```python
from build123d import *

# Parameters (mm, degrees)
SKETCH1_R           = 15.24
SKETCH1_R_2         = 4.55
BOSS_EXTRUDE1_DEPTH = 2.54
SKETCH2_R           = 5.95
BOSS_EXTRUDE2_DEPTH = 7
BOSS_EXTRUDE3_DEPTH = 38.1
SKETCH5_R           = 0.9525
BOSS_EXTRUDE5_DEPTH = 2.54


with BuildPart() as part:
    # Sketch1 → Boss-Extrude1 (new body)
    with BuildSketch(Plane.XY):
        Circle(SKETCH1_R)
        Circle(SKETCH1_R_2, mode=Mode.SUBTRACT)
    extrude(amount=BOSS_EXTRUDE1_DEPTH)

    # Sketch2 → Boss-Extrude2 (add)
    with BuildSketch(Plane.XY.offset(2.54)):
        Circle(SKETCH2_R)
    extrude(amount=BOSS_EXTRUDE2_DEPTH)

    # Sketch3 → Boss-Extrude3 (add)
    with BuildSketch(Plane.XY.offset(9.54)):
        Polygon((3.666174209, 6.35), (-3.666174209, 6.35), (-7.332348419, 0), (-3.666174209, -6.35), (3.666174209, -6.35), (7.332348419, 0), align=None)
    extrude(amount=BOSS_EXTRUDE3_DEPTH)

    # Sketch5 → Boss-Extrude5 (add)
    with BuildSketch(Plane(origin=(0, 0, 0), x_dir=(-1, 0, 0), z_dir=(0, 0, -1))):
        with Locations(Location((0, 12.7, 0), (0, 0, 180))):
            Circle(SKETCH5_R)
        with Locations(Location((5.165555367, 11.602027312, 0), (0, 0, 180))):
            Circle(SKETCH5_R)
        with Locations(Location((9.437939284, 8.497958701, 0), (0, 0, 180))):
            Circle(SKETCH5_R)
        with Locations(Location((12.078417757, 3.924515829, 0), (0, 0, 180))):
            Circle(SKETCH5_R)
        with Locations(Location((12.630428071, -1.327511483, 0), (0, 0, 180))):
            Circle(SKETCH5_R)
        with Locations(Location((10.998522628, -6.35, 0), (0, 0, 180))):
            Circle(SKETCH5_R)
        with Locations(Location((7.464872704, -10.274515829, 0), (0, 0, 180))):
            Circle(SKETCH5_R)
        with Locations(Location((2.640478473, -12.422474529, 0), (0, 0, 180))):
            Circle(SKETCH5_R)
        with Locations(Location((-2.640478473, -12.422474529, 0), (0, 0, 180))):
            Circle(SKETCH5_R)
        with Locations(Location((-7.464872704, -10.274515829, 0), (0, 0, 180))):
            Circle(SKETCH5_R)
        with Locations(Location((-10.998522628, -6.35, 0), (0, 0, 180))):
            Circle(SKETCH5_R)
        with Locations(Location((-12.630428071, -1.327511483, 0), (0, 0, 180))):
            Circle(SKETCH5_R)
        with Locations(Location((-12.078417757, 3.924515829, 0), (0, 0, 180))):
            Circle(SKETCH5_R)
        with Locations(Location((-9.437939284, 8.497958701, 0), (0, 0, 180))):
            Circle(SKETCH5_R)
        with Locations(Location((-5.165555367, 11.602027312, 0), (0, 0, 180))):
            Circle(SKETCH5_R)
    extrude(amount=BOSS_EXTRUDE5_DEPTH)


solid = part.part
```
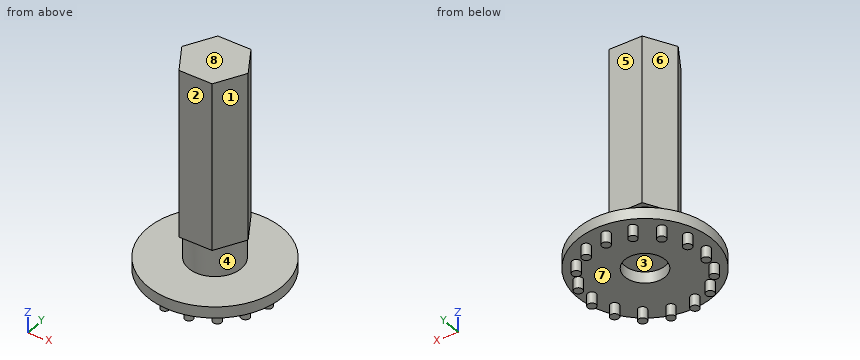
The model under review builds one solid part; all positions refer to its coordinate system, in mm. Face numbers are marked on the shaded views. A direction names the side the tool comes from. Round coordinates to 2 decimals unless told otherwise and drop trailing zeros. Loops run counter-clockwise (first coordinate to the right, second up) from the corner with the lowest first, then second, coordinate; pieces in that order, holes last. Notation, with made-up numbers: (35.25, 22) -> (52.25, 22) arc R15 cw to (52.25, 46) -> close; hole circle Ø4 at (-14, 20). An arc over 180 degrees is marked (long way). Answer as a JSON object with one key per item and string values. Group by question number.
1) We need section A-A on z = 12. Write out the cut boundary in (x, y), then the cut area to 3 significant figures.
2) Mouldability with a two-part tool opening along X and no side actions: class the marked faces 1, 2, 3 and 4 as released by +X, released by -X, zero draft, split by the parting line, or undercut.
3) For line 1 (Y direction, x = 0, z = 0.9); line 2 (Z direction, x = 7, y = 0.5); line 3 (Z direction, x = 9.5, y = -6.5), list the stretches that pass through material, from the lowest coordinate up. Write a range as [from, to].
4) For pin 1 Ø1 at (x, y) = (2, 1) entering from -Z; pin 2 Ø2 at (y, z) = (7, 42.5) entering from -X; pin 3 Ø14 at (x, y) = (3, -3) entering from -Z; pin 4 Ø5 at (y, z) = (0.5, 3) entering from +X, all flat-tipped, find the tip position at first contact; note any pin that passes through.
5) For the marked faces 5, 6, 7 and 8, list the 3-axis set-ups (+Z, -Z, +X, -X, +Y, -Y) from which the entire face can be reached by the end or side of a thin tool; tool diameter is ignored.
6) We need section B-B on y = -3.5. Write out the cut boundary in (x, z).
Result set:
{
 "1": {"outline": "(-7.33, 0) -> (-3.67, -6.35) -> (3.67, -6.35) -> (7.33, 0) -> (3.67, 6.35) -> (-3.67, 6.35) -> close", "area": "140 mm²"},
 "2": {"face 1": "released by +X", "face 2": "zero draft", "face 3": "undercut", "face 4": "split by the parting line"},
 "3": {"line 1": "[-15.24, -4.55], [4.55, 15.24]", "line 2": "[0, 2.54], [9.54, 47.64]", "line 3": "[0, 2.54]"},
 "4": {"pin 1": "z = 2.54", "pin 2": "x = -3.87", "pin 3": "z = 0", "pin 4": "x = 15.24"},
 "5": {"face 5": "+Z, +X, -X, +Y", "face 6": "+Z, -X, +Y", "face 7": "-Z", "face 8": "+Z, +X, -X, +Y, -Y"},
 "6": {"outline": "(-14.83, 0) -> (-2.91, 0) -> (-2.91, 2.54) -> (2.91, 2.54) -> (2.91, 0) -> (14.83, 0) -> (14.83, 2.54) -> (4.81, 2.54) -> (4.81, 9.54) -> (5.31, 9.54) -> (5.31, 47.64) -> (-5.31, 47.64) -> (-5.31, 9.54) -> (-4.81, 9.54) -> (-4.81, 2.54) -> (-14.83, 2.54) -> close"}
}
